from build123d import *

# Parameters (mm, degrees)
EXTRUDE_2_DEPTH     = 12
FILLET_1_R          = 6
CUT_EXTRUDE_1_DEPTH = 0.75
CUT_EXTRUDE_2_REACH = 48.76
SKETCH_4_R          = 4
CUT_EXTRUDE_3_REACH = 49.366
SKETCH_5_R          = 1.75
CUT_EXTRUDE_4_REACH = 48.76
SKETCH_6_R          = 0.5
EXTRUDE_4_DEPTH     = 1.5


with BuildPart() as part:
    # 草图2 → 凸台-拉伸2 (new body)
    with BuildSketch(Plane(origin=(0, 0, 0), x_dir=(1, 0, 0), z_dir=(0, 1, 0))):
        Polygon((0, 0), (38.4, 0), (38.4, 25), (36.9, 25), (36.9, 1.5), (1.5, 1.5), (1.5, 25), (0, 25), align=None)
    extrude(amount=EXTRUDE_2_DEPTH)

    # 圆角1
    fillet_1_edges = [part.edges().sort_by_distance(p)[0] for p in [
        (0.75, 0, -25),
        (0.75, 12, -25),
        (37.65, 0, -25),
        (37.65, 12, -25),
    ]]
    fillet(fillet_1_edges, radius=FILLET_1_R - 0.0001)  # a hair under: the kernel refuses the full size

    # 草图3 → 切除-拉伸1 (cut)
    with BuildSketch(Plane(origin=(38.4, 0, 0), x_dir=(0, 0, -1), z_dir=(1, 0, 0))):
        with BuildLine():
            Line((18.542857143, 9.973791692), (4.725714286, 8.384275015))
            ThreePointArc((4.725714286, 8.384275015), (2.6, 6), (4.725714286, 3.615724985))
            Line((4.725714286, 3.615724985), (18.542857143, 2.026208308))
            ThreePointArc((18.542857143, 2.026208308), (23, 6), (18.542857143, 9.973791692))
        make_face()
    extrude(amount=-CUT_EXTRUDE_1_DEPTH, mode=Mode.SUBTRACT)

    # 草图4 → 切除-拉伸2 (cut, up to next)
    with BuildSketch(Plane(origin=(37.65, 0, 0), x_dir=(0, 0, -1), z_dir=(1, 0, 0)), mode=Mode.PRIVATE) as cut_extrude_2_sk1:
        with Locations((19, 6)):
            Circle(SKETCH_4_R)
    cut_extrude_2_tool1 = extrude(cut_extrude_2_sk1.sketch, amount=-CUT_EXTRUDE_2_REACH, mode=Mode.PRIVATE) & part.part
    add(cut_extrude_2_tool1.solids().sort_by_distance((37.65, 6, -19))[0], mode=Mode.SUBTRACT)

    # 草图5 → 切除-拉伸3 (cut, up to next)
    with BuildSketch(Plane.ZY, mode=Mode.PRIVATE) as cut_extrude_3_sk1:
        with Locations((-19, 6)):
            Circle(SKETCH_5_R)
    cut_extrude_3_tool1 = extrude(cut_extrude_3_sk1.sketch, amount=-CUT_EXTRUDE_3_REACH, mode=Mode.PRIVATE) & part.part
    add(cut_extrude_3_tool1.solids().sort_by_distance((0, 6, -19))[0], mode=Mode.SUBTRACT)

    # 草图6 → 切除-拉伸4 (cut, up to next)
    with BuildSketch(Plane(origin=(37.65, 0, 0), x_dir=(0, 0, -1), z_dir=(1, 0, 0)), mode=Mode.PRIVATE) as cut_extrude_4_sk1:
        with Locations((8.5, 6)):
            Circle(SKETCH_6_R)
    cut_extrude_4_tool1 = extrude(cut_extrude_4_sk1.sketch, amount=-CUT_EXTRUDE_4_REACH, mode=Mode.PRIVATE) & part.part
    add(cut_extrude_4_tool1.solids().sort_by_distance((37.65, 6, -8.5))[0], mode=Mode.SUBTRACT)

    # 草图7 → 凸台-拉伸4 (add)
    with BuildSketch(Plane(origin=(38.4, 0, 0), x_dir=(0, 0, -1), z_dir=(1, 0, 0))):
        with BuildLine():
            Line((19, 12), (20.986136983, 14.836497573))
            ThreePointArc((20.986136983, 14.836497573), (21.882023258, 15.140609984), (22.441458618, 14.377636424))
            Line((22.441458618, 14.377636424), (22.441458618, 10.914912266))
            ThreePointArc((22.441458618, 10.914912266), (20.804234797, 11.722301704), (19, 12))
        make_face()
        with BuildLine():
            Line((26.729122981, 10.721132005), (24.681580777, 7.928636792))
            ThreePointArc((24.681580777, 7.928636792), (23.838667626, 9.54785789), (22.54785789, 10.838667626))
            Line((22.54785789, 10.838667626), (25.826815726, 11.951723827))
            ThreePointArc((25.826815726, 11.951723827), (26.729122981, 11.667227443), (26.729122981, 10.721132005))
        make_face()
        with BuildLine():
            Line((28.02476043, 5.237026439), (24.722301704, 4.195765203))
            ThreePointArc((24.722301704, 4.195765203), (25, 6), (24.722301704, 7.804234797))
            Line((24.722301704, 7.804234797), (28.02476043, 6.762973561))
            ThreePointArc((28.02476043, 6.762973561), (28.58419579, 6), (28.02476043, 5.237026439))
        make_face()
        with BuildLine():
            Line((25.826815726, 0.048276173), (22.54785789, 1.161332374))
            ThreePointArc((22.54785789, 1.161332374), (23.838667626, 2.45214211), (24.681580777, 4.071363208))
            Line((24.681580777, 4.071363208), (26.729122981, 1.278867995))
            ThreePointArc((26.729122981, 1.278867995), (26.729122981, 0.332772557), (25.826815726, 0.048276173))
        make_face()
        with BuildLine():
            Line((20.986136983, -2.836497573), (19, 0))
            ThreePointArc((19, 0), (20.804234797, 0.277698296), (22.441458618, 1.085087734))
            Line((22.441458618, 1.085087734), (22.441458618, -2.377636424))
            ThreePointArc((22.441458618, -2.377636424), (21.882023258, -3.140609984), (20.986136983, -2.836497573))
        make_face()
    extrude(amount=-EXTRUDE_4_DEPTH)


solid = part.part
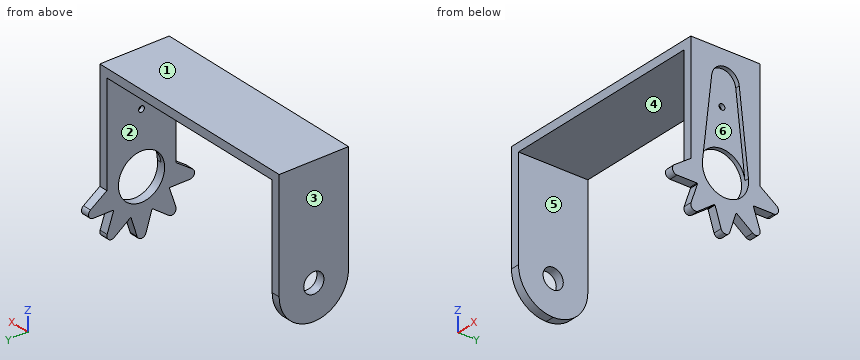
Could you check a few things on this model? Use its own coordinates, in mm. Face numbers are marked on the shaded views. A direction names the side the tool comes from. Coordinates: 2 decimals unless noted, no trailing zeros. Order: outer loops, then holes, each group sorted by start corner. A loop starts at its lowest first (then second) coordinate and runs counter-clockwise, first axis right, second up. Notation, with made-up numbers: (6, 89) -> (54, 89) arc R19 cw to (54, 123) -> close; hole circle Ø8 at (10, 21.25). An arc over 180 degrees is marked (long way). One line per item, written item: value. Start each with the question number.
1) If I drill on L1, parallel to X at y = 6.75, z = -14.75; L2, parallel to Y at x = 37.3, z = -8.5; L3, parallel to X at y = 10, z = -19.5, over which ranges is the centre line in solid material (lowest first)? Write a range as [from, to].
2) Which directions (+Z, -Z, +X, -X, +Y, -Y) give clear straight access to the entire face, cutting with the end or side of a thin tool? Please do the marked faces 1 and 2.
3) Imagine slicing it at A-A on z = -4. List the corners of the cut face in (x, y) for me, plus the area to 3 significant figures.
4) We'd pull the mould along X, two halves only. Please class the marked faces 3, 4, 5 and 6: +X half, -X half, draft (parallel to the pull), parting line (faces both ways), or undercut.
5) Imagine slicing it at B-B on z = -8.5. List the corners of the cut face in (x, y) for me, plus the area to 3 significant figures.
6) I'm going to push flat-ended pins straight in: pin 1 (10 mm diameter, centred on x = 7.5, y = 11, fed in from -Z); pin 2 (1 mm diameter, centred on y = 6.5, z = -12, fed in from +X); pin 3 (6.5 mm diameter, centred on y = 6, z = -19, fed in from +X); pin 4 (2 mm diameter, centred on y = 6, z = -19, fed in from -X). Where does each tip first touch, or does it pass through?
7) Imagine slicing it at C-C on y = 2.5. List the corners of the cut face in (x, z) for me.
8) Imagine slicing it at D-D on x = 13.5. List the corners of the cut face in (y, z) for me.
Answer list:
1. L1: x = [0, 1.5], [36.9, 37.65]
1. L2: y = [0, 5.5], [6.5, 12]
1. L3: x = [0, 1.5], [36.9, 38.4]
2. face 1: +Z, +X, -X, +Y, -Y
2. face 2: -Z, +Y, -Y
3. outline: (0, 0) -> (1.5, 0) -> (1.5, 12) -> (0, 12) -> close; (36.9, 0) -> (38.4, 0) -> (38.4, 3.82) -> (37.65, 3.82) -> (37.65, 8.18) -> (38.4, 8.18) -> (38.4, 12) -> (36.9, 12) -> close
3. area: 32.7 mm2
4. face 3: -X half
4. face 4: undercut
4. face 5: undercut
4. face 6: +X half
5. outline: (0, 0) -> (1.5, 0) -> (1.5, 12) -> (0, 12) -> close; (36.9, 0) -> (38.4, 0) -> (38.4, 3.18) -> (37.65, 3.18) -> (37.65, 5.5) -> (36.9, 5.5) -> close; (36.9, 6.5) -> (37.65, 6.5) -> (37.65, 8.82) -> (38.4, 8.82) -> (38.4, 12) -> (36.9, 12) -> close
5. area: 31.0 mm2
6. pin 1: stops at z = -1.5
6. pin 2: stops at x = 37.65
6. pin 3: stops at x = 1.5
6. pin 4: passes through
7. outline: (0, -23.87) -> (1.5, -23.87) -> (1.5, -1.5) -> (36.9, -1.5) -> (36.9, -17.06) -> (37.65, -17.06) -> (37.65, -14.42) -> (38.4, -14.42) -> (38.4, 0) -> (0, 0) -> close; (36.9, -25.83) -> (38.4, -25.83) -> (38.4, -20.94) -> (36.9, -20.94) -> close
8. outline: (0, -1.5) -> (12, -1.5) -> (12, 0) -> (0, 0) -> close
